```python
from build123d import *

# Parameters (mm, degrees)
SKETCH1_R           = 15
BOSS_EXTRUDE1_DEPTH = 15
SKETCH2_R           = 20
BOSS_EXTRUDE2_DEPTH = 10
SKETCH3_W           = 40
SKETCH3_H           = 40
BOSS_EXTRUDE3_DEPTH = 20
SKETCH4_W           = 80
SKETCH4_H           = 40
BOSS_EXTRUDE4_DEPTH = 10
SKETCH5_W           = 4.531505326
SKETCH5_H           = 40
BOSS_EXTRUDE5_DEPTH = 20


with BuildPart() as part:
    # Sketch1 → Boss-Extrude1 (new, symmetric)
    with BuildSketch(Plane.XY):
        Circle(SKETCH1_R)
    extrude(amount=BOSS_EXTRUDE1_DEPTH, both=True)

    # Sketch2 → Boss-Extrude2 (add)
    with BuildSketch(Plane(origin=(0, 0, -15), x_dir=(-1, 0, 0), z_dir=(0, 0, -1))):
        Circle(SKETCH2_R)
    extrude(amount=BOSS_EXTRUDE2_DEPTH)

    # Sketch3 → Boss-Extrude3 (add)
    with BuildSketch(Plane.XY.offset(15)):
        Rectangle(SKETCH3_W, SKETCH3_H)
    extrude(amount=BOSS_EXTRUDE3_DEPTH)

    # Sketch4 → Boss-Extrude4 (add)
    with BuildSketch(Plane.XY.offset(35)):
        Rectangle(SKETCH4_W, SKETCH4_H)
    extrude(amount=BOSS_EXTRUDE4_DEPTH)

    # Sketch5 → Boss-Extrude5 (add)
    with BuildSketch(Plane.XY.offset(45)):
        with Locations((-19.705182252, 0)):
            Rectangle(SKETCH5_W, SKETCH5_H)
    boss_extrude5 = extrude(amount=BOSS_EXTRUDE5_DEPTH)

    # Mirror1: Boss-Extrude5 across plane
    add(boss_extrude5.mirror(Plane(origin=(0, 0, 0), x_dir=(0, 0, 1), z_dir=(1, 0, 0))))


solid = part.part
```
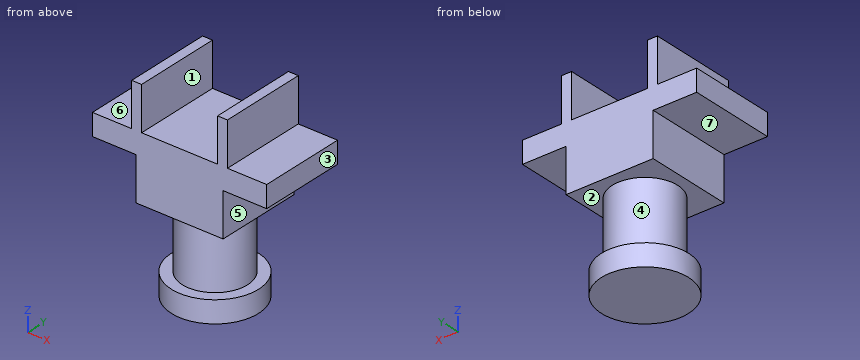
The model under review builds one solid part; all positions refer to its coordinate system, in mm. Face numbers are marked on the shaded views. A direction names the side the tool comes from. Round coordinates to 2 decimals unless told otherwise and drop trailing zeros. Loops run counter-clockwise (first coordinate to the right, second up) from the corner with the lowest first, then second, coordinate; pieces in that order, holes last. Notation, with made-up numbers: (28, 88.25) - (45, 88.25) arc R23 ccw to (45, 113.25) - close; hole circle Ø5 at (-7, 26). An arc over 180 degrees is marked (long way). Use a Markdown table: item, result. Add a question column.
Q1. For probe 1 along Z at (x, y) = (8.5, 17); probe 2 along X at (y, z) = (-10.5, 51); probe 3 along Z at (x, y) = (-11.5, -16.5), list the stretches that pass through material, from the lowest coordinate up.
Q2. Add section A-A (x = 0). State the section outline as (y, z) points.
Q3. Add section C-C (y = 0). State the section outline as (x, z) points.
Q4. Insertion check: pin 1 Ø12 at (y, z) = (12, 53.5) entering from +X; pin 2 Ø16 at (x, y) = (32, -8.5) entering from -Z; pin 3 Ø22 at (y, z) = (9, 22) entering from +X. Each pin has a flat end and moves straight along its axis. Give the tip position at first contact, or say it passes through.
Q5. Add section B-B (y = 17). State the section outline as (x, z) points, plus the area to 3 significant figures.
Q6. The part is to be moulded in two halves that separate along X. For the marked faces 1, 2, 3 and 4, say which applies: pulls with the +X half, pulls with the -X half, needs draft (parallel to the pull), parting line crosses it, or undercut.
Q7. Add section D-D (z = 22). State the section outline as (x, y) points, plus the area to 3 significant figures.
Q8. Machinability: for the marked faces 5, 6 and 7, which of the approach directions +Z, -Z, +X, -X, +Y, -Y give a long, thin tool a straight path to every point of the face, cutting with its end or side? Answer none if there is none.
Worked answers:
| question | item | result |
|---|---|---|
| 1 | probe 1 | -25 to -15, 15 to 45 |
| 1 | probe 2 | -21.97 to -17.44, 17.44 to 21.97 |
| 1 | probe 3 | 15 to 45 |
| 2 | outline | (-20, -25) - (20, -25) - (20, -15) - (15, -15) - (15, 15) - (20, 15) - (20, 45) - (-20, 45) - (-20, 15) - (-15, 15) - (-15, -15) - (-20, -15) - close |
| 3 | outline | (-40, 35) - (-20, 35) - (-20, 15) - (-15, 15) - (-15, -15) - (-20, -15) - (-20, -25) - (20, -25) - (20, -15) - (15, -15) - (15, 15) - (20, 15) - (20, 35) - (40, 35) - (40, 45) - (21.97, 45) - (21.97, 65) - (17.44, 65) - (17.44, 45) - (-17.44, 45) - (-17.44, 65) - (-21.97, 65) - (-21.97, 45) - (-40, 45) - close |
| 4 | pin 1 | x = 21.97 |
| 4 | pin 2 | z = 35 |
| 4 | pin 3 | x = 20 |
| 5 | outline | (-40, 35) - (-20, 35) - (-20, 15) - (20, 15) - (20, 35) - (40, 35) - (40, 45) - (21.97, 45) - (21.97, 65) - (17.44, 65) - (17.44, 45) - (-17.44, 45) - (-17.44, 65) - (-21.97, 65) - (-21.97, 45) - (-40, 45) - close; (-10.54, -25) - (10.54, -25) - (10.54, -15) - (-10.54, -15) - close |
| 5 | area | 1,990 mm² |
| 6 | face 1 | undercut |
| 6 | face 2 | needs draft |
| 6 | face 3 | pulls with the +X half |
| 6 | face 4 | parting line crosses it |
| 7 | outline | (-20, -20) - (20, -20) - (20, 20) - (-20, 20) - close |
| 7 | area | 1,600 mm² |
| 8 | face 5 | -Z, +X, +Y, -Y |
| 8 | face 6 | +Z, -X, +Y, -Y |
| 8 | face 7 | -Z, -X, +Y, -Y |
